```python
from build123d import *

# Parameters (mm, degrees)
ESQUISSE1_W                                      = 80
ESQUISSE1_H                                      = 80
ESQUISSE1_R                                      = 27
BOSS_EXTRU_1_DEPTH                               = 15
CHAMBRAGE_POUR_VIS_T_TE_CYLINDRIQUE_D            = 4.5
CHAMBRAGE_POUR_VIS_T_TE_CYLINDRIQUE_CBORE_D      = 8
CHAMBRAGE_POUR_VIS_T_TE_CYLINDRIQUE_CBORE_DEPTH  = 7
CHAMBRAGE_POUR_VIS_T_TE_CYLINDRIQU_2_D           = 4.5
CHAMBRAGE_POUR_VIS_T_TE_CYLINDRIQU_2_CBORE_D     = 8
CHAMBRAGE_POUR_VIS_T_TE_CYLINDRIQU_2_CBORE_DEPTH = 7
R_P_TITION_CIRCULAIRE3_COUNT                     = 4
ESQUISSE2_W                                      = 80
ESQUISSE2_H                                      = 60
BOSS_EXTRU_2_DEPTH                               = 15
TROU_TARAUD_PROFOND_M5X0_81_AT_2_COUNT           = 2
TROU_TARAUD_PROFOND_M5X0_81_AT_2_PITCH           = 20
TROU_TARAUD_M6X1_01_D                            = 5
R_P_TITION_LIN_AIRE1_COUNT                       = 2
R_P_TITION_LIN_AIRE1_PITCH                       = 25
TROU_TARAUD_M5X0_81_D                            = 4.2
R_P_TITION_CIRCULAIRE2_COUNT                     = 4


with BuildPart() as part:
    # Esquisse1 → Boss.-Extru.1 (new body)
    with BuildSketch(Plane.XY):
        Rectangle(ESQUISSE1_W, ESQUISSE1_H)
        Circle(ESQUISSE1_R, mode=Mode.SUBTRACT)
    extrude(amount=BOSS_EXTRU_1_DEPTH)

    # Chambrage pour vis _ t_te cylindrique (through all)
    with Locations(Plane(origin=(31.5, 31.5, 15), x_dir=(1, 0, 0), z_dir=(0, 0, 1))):
        with Locations((0, 0)):
            chambrage_pour_vis_t_te_cylindrique = CounterBoreHole(CHAMBRAGE_POUR_VIS_T_TE_CYLINDRIQUE_D / 2, CHAMBRAGE_POUR_VIS_T_TE_CYLINDRIQUE_CBORE_D / 2, CHAMBRAGE_POUR_VIS_T_TE_CYLINDRIQUE_CBORE_DEPTH)

    # Chambrage pour vis _ t_te cylindriqu 2 (through all)
    with Locations(Plane(origin=(22.980970389, 22.980970389, 0), x_dir=(-1, 0, 0), z_dir=(0, 0, -1))):
        with Locations((0, 0)):
            chambrage_pour_vis_t_te_cylindriqu_2 = CounterBoreHole(CHAMBRAGE_POUR_VIS_T_TE_CYLINDRIQU_2_D / 2, CHAMBRAGE_POUR_VIS_T_TE_CYLINDRIQU_2_CBORE_D / 2, CHAMBRAGE_POUR_VIS_T_TE_CYLINDRIQU_2_CBORE_DEPTH)

    # Répétition circulaire3: Chambrage pour vis _ t_te cylindrique, Chambrage pour vis _ t_te cylindriqu 2 ×4 about axis
    r_p_tition_circulaire3_axis = Axis((0, 0, 0), (0, 0, 1))
    add([chambrage_pour_vis_t_te_cylindrique.rotate(r_p_tition_circulaire3_axis, i * 360 / R_P_TITION_CIRCULAIRE3_COUNT) for i in range(1, R_P_TITION_CIRCULAIRE3_COUNT)], mode=Mode.SUBTRACT)
    add([chambrage_pour_vis_t_te_cylindriqu_2.rotate(r_p_tition_circulaire3_axis, i * 360 / R_P_TITION_CIRCULAIRE3_COUNT) for i in range(1, R_P_TITION_CIRCULAIRE3_COUNT)], mode=Mode.SUBTRACT)

    # Esquisse2 → Boss.-Extru.2 (add)
    with BuildSketch(Plane.XY.offset(15)):
        with Locations((0, 70)):
            Rectangle(ESQUISSE2_W, ESQUISSE2_H)
    extrude(amount=-BOSS_EXTRU_2_DEPTH)

    # Esquisse10 → Trou taraudé profond M5x0.81 (revolve, cut)
    with BuildSketch(Plane(origin=(40, 55, 7.5), x_dir=(0, 0, -1), z_dir=(0, 1, 0))):
        Polygon((0, 0), (0, 23.6618073), (2.1, 22.4), (2.1, 0), align=None)
    trou_taraud_profond_m5x0_81 = revolve(axis=Axis((46.35, 55, 7.5), (-1, 0, 0)), mode=Mode.SUBTRACT)

    # Trou taraudé profond M5x0.81 at 2: Trou taraudé profond M5x0.81 ×2
    with Locations(*[(0, i * TROU_TARAUD_PROFOND_M5X0_81_AT_2_PITCH, 0) for i in range(1, TROU_TARAUD_PROFOND_M5X0_81_AT_2_COUNT)]):
        add(trou_taraud_profond_m5x0_81, mode=Mode.SUBTRACT)

    # Symétrie1: Trou taraudé profond M5x0.81 across plane
    add(trou_taraud_profond_m5x0_81.mirror(Plane(origin=(0, 0, 0), x_dir=(0, 0, 1), z_dir=(1, 0, 0))), mode=Mode.SUBTRACT)

    # Symétrie1 copy 1 sketch → Symétrie1 copy 1 (revolve, cut)
    with BuildSketch(Plane(origin=(-40, 75, 7.5), x_dir=(0, 0, -1), z_dir=(0, 1, 0))):
        Polygon((0, 0), (0, -23.6618073), (2.1, -22.4), (2.1, 0), align=None)
    revolve(axis=Axis((-46.35, 75, 7.5), (-1, 0, 0)), mode=Mode.SUBTRACT)

    # Trou taraudé M6x1.01 (through all)
    with Locations(Plane(origin=(-25, 90, 15), x_dir=(1, 0, 0), z_dir=(0, 0, 1))):
        with Locations((0, 0), (25, 0), (50, 0)):
            trou_taraud_m6x1_01 = Hole(TROU_TARAUD_M6X1_01_D / 2)

    # Répétition linéaire1: Trou taraudé M6x1.01 ×2
    with Locations(*[(0, -i * R_P_TITION_LIN_AIRE1_PITCH, 0) for i in range(1, R_P_TITION_LIN_AIRE1_COUNT)]):
        add(trou_taraud_m6x1_01, mode=Mode.SUBTRACT)

    # Trou taraudé M5x0.81 (through all)
    with Locations(Plane(origin=(-32.75, 0, 15), x_dir=(1, 0, 0), z_dir=(0, 0, 1))):
        with Locations((0, 0)):
            trou_taraud_m5x0_81 = Hole(TROU_TARAUD_M5X0_81_D / 2)

    # Répétition circulaire2: Trou taraudé M5x0.81 ×4 about axis
    r_p_tition_circulaire2_axis = Axis((0, 0, 0), (0, 0, 1))
    for i in range(1, R_P_TITION_CIRCULAIRE2_COUNT):
        add(trou_taraud_m5x0_81.rotate(r_p_tition_circulaire2_axis, i * 360 / R_P_TITION_CIRCULAIRE2_COUNT), mode=Mode.SUBTRACT)


solid = part.part
```
Build history of the part. All positions in model axes, mm. A direction names the side the tool comes from. Coordinates: 2 decimals unless noted, no trailing zeros. Order: outer loops, then holes, each group sorted by start corner. A loop starts at its lowest first (then second) coordinate and runs counter-clockwise, first axis right, second up.
Item 1: Mould opens along Y. For faces 4 (the flat face through (-1, -40, 7)), 5 (the cylindrical face through (-28.957, 76.278, 9.166)) say: released by +Y, released by -Y, zero draft, split by the parting line, or undercut.
Filled in:
face 4: released by -Y
face 5: undercut
Item 2: Saw through at C-C on z = 2.25. State how many separate pieces and enclosed holes the cut face has, then the cut area to 3 significant figures.
Filled in:
separate pieces: 1
enclosed holes: 19
area: 8,470 mm2
Item 3: Tool access for faces 1 (the cylindrical face through (-20.831, -26.354, 3.451)), 2 (the cylindrical face through (28.96, 57.05, 7.96)), 3 (the flat face through (-29.8, 33.2, 8)): list every direction of +Z, -Z, +X, -X, +Y, -Y with a clear straight run to the whole face (end or side of a thin tool).
Filled in:
face 1: -Z
face 2: +X
face 3: +Z
Item 4: Drop flat-ended pins along their axis: pin 1 Ø5 at (y, z) = (75, 7.5) entering from -X; pin 2 Ø3.5 at (y, z) = (55, 7.5) entering from -X; pin 3 Ø6.5 at (x, y) = (-31, -31.5) entering from +Z; pin 4 Ø7 at (x, y) = (-22.98, 22.98) entering from -Z. Give the stop position or say it passes through.
Filled in:
pin 1: stops at x = -40
pin 2: stops at x = -17.39
pin 3: stops at z = 8
pin 4: stops at z = 7
Item 5: Saw through at B-B on x = 0. List the corners of the cut face in (y, z).
Filled in:
outline: (-40, 0) - (-34.85, 0) - (-34.85, 15) - (-40, 15) - close; (-30.65, 0) - (-27, 0) - (-27, 15) - (-30.65, 15) - close; (27, 0) - (30.65, 0) - (30.65, 15) - (27, 15) - close; (34.85, 0) - (62.5, 0) - (62.5, 15) - (34.85, 15) - close; (67.5, 0) - (87.5, 0) - (87.5, 15) - (67.5, 15) - close; (92.5, 0) - (100, 0) - (100, 15) - (92.5, 15) - close
Item 6: Drill centre lines: L1, parallel to Y at x = 22, z = 12.5; L2, parallel to Z at x = 23.75, y = 75; L3, parallel to X at y = 24, z = 8. Where is each one in solid material? Low to high.
Filled in:
L1: y = -40 to -25.01, -20.96 to -15.65, 15.65 to 20.96, 25.01 to 100
L2: z = 0 to 5.4, 9.6 to 15
L3: x = -40 to -24.99, -20.97 to -12.37, 12.37 to 20.97, 24.99 to 40
Item 7: Saw through at D-D on x = 11. List the corners of the cut face in (y, z).
Filled in:
outline: (-40, 0) - (-24.66, 0) - (-24.66, 15) - (-40, 15) - close; (24.66, 0) - (100, 0) - (100, 15) - (24.66, 15) - close
Item 8: Saw through at A-A on y = 90. List the corners of the cut face in (x, z), then the cut area to 3 significant figures.
Filled in:
outline: (-40, 0) - (-27.5, 0) - (-27.5, 15) - (-40, 15) - close; (-22.5, 0) - (-2.5, 0) - (-2.5, 15) - (-22.5, 15) - close; (2.5, 0) - (22.5, 0) - (22.5, 15) - (2.5, 15) - close; (27.5, 0) - (40, 0) - (40, 15) - (27.5, 15) - close
area: 975 mm2
